Design review of the part built by this model. Coordinates are the model's own, in mm. Coordinates: 2 decimals unless noted, no trailing zeros. Loops run counter-clockwise (first coordinate to the right, second up) from the corner with the lowest first, then second, coordinate; pieces in that order, holes last. Notation, with made-up numbers: (26.25, 11.5) -> (46.25, 11.5) arc R17 ccw to (46.25, 16.5) -> close; hole circle Ø2 at (59.25, 79). An arc over 180 degrees is marked (long way). Use CSV: the item, a comma, the result in double quotes.
```python
from build123d import *

# Parameters (mm, degrees)
BOSS_EXTRUDE1_DEPTH = 3


with BuildPart() as part:
    # Sketch1 → Boss-Extrude1 (new body)
    with BuildSketch(Plane(origin=(0, 0, 0), x_dir=(1, 0, 0), z_dir=(0, 1, 0))):
        with BuildLine():
            Line((-62.418566214, -48.6586621), (-58.418566214, -48.6586621))
            Line((-58.418566214, -48.6586621), (-58.418566214, -38.1586621))
            Line((-58.418566214, -38.1586621), (-48.418566214, -38.1586621))
            Line((-48.418566214, -38.1586621), (-48.418566214, -48.6586621))
            Line((-48.418566214, -48.6586621), (-44.418566214, -48.6586621))
            Line((-44.418566214, -48.6586621), (-43.418817081, -58.656153425))
            Line((-43.418817081, -58.656153425), (-43.418817081, -60.6586621))
            Line((-43.418817081, -60.6586621), (-40.418817081, -60.6586621))
            Line((-40.418817081, -60.6586621), (-40.418817081, -58.6586621))
            Line((-40.418817081, -58.6586621), (-38.722684913, -53.544656797))
            ThreePointArc((-38.722684913, -53.544656797), (-37.43326006, -52.606013311), (-36.129099744, -53.524073178))
            Line((-36.129099744, -53.524073178), (-34.335191263, -58.6586621))
            Line((-34.335191263, -58.6586621), (28.581433786, -58.6586621))
            Line((28.581433786, -58.6586621), (28.581433786, -60.6586621))
            Line((28.581433786, -60.6586621), (31.581433786, -60.6586621))
            Line((31.581433786, -60.6586621), (31.581433786, -58.708800497))
            Line((31.581433786, -58.708800497), (32.581433786, -48.711334262))
            Line((32.581433786, -48.711334262), (36.581433786, -48.711334262))
            Line((36.581433786, -48.711334262), (36.581433786, -38.211334262))
            Line((36.581433786, -38.211334262), (46.581433786, -38.211334262))
            Line((46.581433786, -38.211334262), (46.581433786, -48.711334262))
            Line((46.581433786, -48.711334262), (50.581433786, -48.711334262))
            Line((50.581433786, -48.711334262), (41.830582941, -63.6586621))
            Line((41.830582941, -63.6586621), (-53.758312176, -63.6586621))
            Line((-53.758312176, -63.6586621), (-60.382083638, -58.930990881))
            ThreePointArc((-60.382083638, -58.930990881), (-60.567785948, -58.371516574), (-60.091610782, -58.024019727))
            Line((-60.091610782, -58.024019727), (-59.609550678, -58.024019727))
            ThreePointArc((-59.609550678, -58.024019727), (-58.310512573, -57.274019727), (-58.310512573, -55.774019727))
            Line((-58.310512573, -55.774019727), (-62.418566214, -48.6586621))
        make_face()
        Polygon((36.547763078, -52.711334262), (39.581433786, -52.711334262), (39.581433786, -44.211334262), (39.581433786, -41.211334262), (43.581433786, -41.211334262), (43.581433786, -44.211334262), (43.604572315, -52.711334262), (40.093380681, -58.708800497), (35.947864455, -58.708800497), align=None, mode=Mode.SUBTRACT)
        Polygon((-55.418566214, -41.1586621), (-51.418566214, -41.1586621), (-51.418566214, -44.1586621), (-51.418566214, -52.6586621), (-48.038516462, -52.6586621), (-47.438516462, -58.6586621), (-52.026261368, -58.6586621), (-55.490362984, -52.6586621), (-55.418566214, -44.1586621), align=None, mode=Mode.SUBTRACT)
    extrude(amount=BOSS_EXTRUDE1_DEPTH)


solid = part.part
```
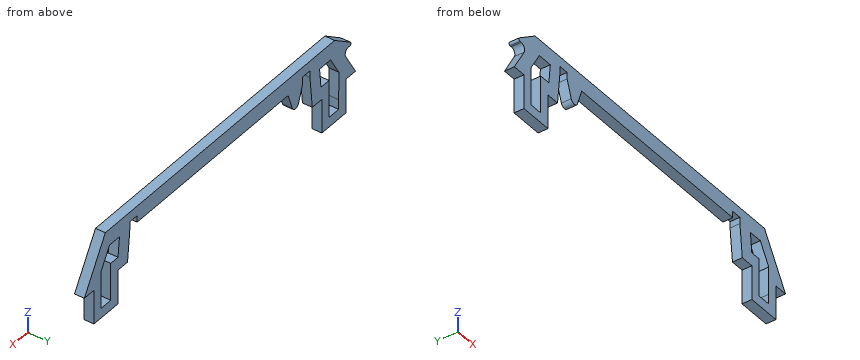
Item 1: Clearance check with flat-ended pins moving along their axes: pin 1 (1.5 mm diameter, centred on x = -54, y = 1.5, fed in from +Z); pin 2 (1.5 mm diameter, centred on y = 2.5, z = 51, fed in from -X); pin 3 (1.5 mm diameter, centred on y = 2, z = 42, fed in from -X); pin 4 (1 mm diameter, centred on y = 2, z = 59.5, fed in from -X). State where each tip first meets the part, or that it passes through.
Checked values:
pin 1,"z = 63.66"
pin 2,"x = -61.5"
pin 3,"x = -58.42"
pin 4,"x = -60.29"
Item 2: Add section B-B (y = 2.5). State how many separate pieces and enclosed holes the cut face has, then the cut area to 3 significant figures.
Checked values:
separate pieces,"1"
enclosed holes,"2"
area,"878 mm^2"
Item 3: Add section A-A (z = 42.25). Give the boundary of the cut face in (x, y), then the cut area to 3 significant figures.
Checked values:
outline,"(-58.42, 0) -> (-55.42, 0) -> (-55.42, 3) -> (-58.42, 3) -> close; (-51.42, 0) -> (-48.42, 0) -> (-48.42, 3) -> (-51.42, 3) -> close; (36.58, 0) -> (39.58, 0) -> (39.58, 3) -> (36.58, 3) -> close; (43.58, 0) -> (46.58, 0) -> (46.58, 3) -> (43.58, 3) -> close"
area,"36.0 mm^2"
Item 4: Add section C-C (x = -28). Give the boundary of the cut face in (y, z), then the cut area to 3 significant figures.
Checked values:
outline,"(0, 58.66) -> (3, 58.66) -> (3, 63.66) -> (0, 63.66) -> close"
area,"15.0 mm^2"
Item 5: To check wall thickness, follow line 1 along X through (y, z) = (1.95, 42.25); line 2 along Z through (x, y) = (-48.5, 0.75); line 3 along X through (y, z) = (2.6, 50). State the ranges of each line that lie inside material, in increasing order.
Checked values:
line 1,"-58.42 to -55.42, -51.42 to -48.42, 36.58 to 39.58, 43.58 to 46.58"
line 2,"38.16 to 52.66, 58.66 to 63.66"
line 3,"-61.64 to -55.47, -51.42 to -44.28, 32.45 to 39.58, 43.6 to 49.83"
